from build123d import *

# Parameters (mm, degrees)
F0_W     = 37
F0_H     = 10
F0_R     = 1.5
F1_DEPTH = 11
F2_W     = 3.5
F2_H     = 11
F3_DEPTH = 16
F4_W     = 28
F4_H     = 10
F5_DEPTH = 6
F6_DEPTH = 7.5
F7_DEPTH = 7.5
F8_R     = 1
F9_DEPTH = 4
F10_R    = 5.2
F11_R    = 5.7


with BuildPart() as f1:
    # F0 (on Front) → F1 (new body)
    with BuildSketch(Plane.XZ):
        with Locations((-18.5, 5)):
            Rectangle(F0_W, F0_H)
        with Locations((-13.5, 5)):
            Circle(F0_R, mode=Mode.SUBTRACT)
        with Locations((-5, 5)):
            Circle(F0_R, mode=Mode.SUBTRACT)
    extrude(amount=-F1_DEPTH)

    # F2 (on face) → F3 (join)
    with BuildSketch(Plane.XY.offset(10)):
        with Locations((-35.25, 5.5)):
            Rectangle(F2_W, F2_H)
    extrude(amount=F3_DEPTH)

    # F4 (on face) → F5 (cut)
    with BuildSketch(Plane(origin=(0, 11, 0), x_dir=(-1, 0, 0), z_dir=(0, 1, 0))):
        with Locations((14, 5)):
            Rectangle(F4_W, F4_H)
        Polygon((6.5877132403, 7.75), (8.1754264805, 5), (6.5877132403, 2.25), (3.4122867597, 2.25), (1.8245735195, 5), (3.4122867597, 7.75), align=None, mode=Mode.SUBTRACT)
        Polygon((16.6754264805, 5), (15.0877132403, 2.25), (11.9122867597, 2.25), (10.3245735195, 5), (11.9122867597, 7.75), (15.0877132403, 7.75), align=None, mode=Mode.SUBTRACT)
    extrude(amount=-F5_DEPTH, mode=Mode.SUBTRACT)

    # F6 (cut): a face of the model
    f6_faces = [f1.faces().sort_by_distance(p)[0] for p in [
        (-2.6911883006, 11, 3.6670069439),
    ]]
    extrude(f6_faces, amount=-F6_DEPTH, mode=Mode.SUBTRACT)

    # F7 (cut): a face of the model
    f7_faces = [f1.faces().sort_by_distance(p)[0] for p in [
        (-13.5, 11, 7.6659861123),
    ]]
    extrude(f7_faces, amount=-F7_DEPTH, mode=Mode.SUBTRACT)

    # F8 (on face) → F9 (cut)
    with BuildSketch(Plane(origin=(-37, 0, 0), x_dir=(0, -1, 0), z_dir=(-1, 0, 0))):
        with Locations((-8.6, 2)):
            Circle(F8_R)
        with Locations((-2.4, 2)):
            Circle(F8_R)
        with Locations((-2.4, 4.8)):
            Circle(F8_R)
        with Locations((-8.6, 4.8)):
            Circle(F8_R)
        with Locations((-2.4, 7.6)):
            Circle(F8_R)
        with Locations((-8.6, 7.6)):
            Circle(F8_R)
        with Locations((-2.4, 10.4)):
            Circle(F8_R)
        with Locations((-8.6, 10.4)):
            Circle(F8_R)
        with Locations((-2.4, 13.2)):
            Circle(F8_R)
        with Locations((-8.6, 13.2)):
            Circle(F8_R)
        with Locations((-2.4, 16)):
            Circle(F8_R)
        with Locations((-8.6, 16)):
            Circle(F8_R)
        with Locations((-2.4, 18.8)):
            Circle(F8_R)
        with Locations((-8.6, 18.8)):
            Circle(F8_R)
        with Locations((-2.4, 21.6)):
            Circle(F8_R)
        with Locations((-8.6, 21.6)):
            Circle(F8_R)
        with Locations((-2.4, 24.4)):
            Circle(F8_R)
        with Locations((-8.6, 24.4)):
            Circle(F8_R)
    extrude(amount=-F9_DEPTH, mode=Mode.SUBTRACT)

    # F10
    f10_edges = [f1.edges().sort_by_distance(p)[0] for p in [
        (-28, 5, 5),
    ]]
    fillet(f10_edges, radius=F10_R)

    # F11
    f11_edges = [f1.edges().sort_by_distance(p)[0] for p in [
        (-28, 11, 5),
    ]]
    fillet(f11_edges, radius=F11_R)


solid = f1.part
The model under review builds one solid part; all positions refer to its coordinate system, in mm. A direction names the side the tool comes from. Round coordinates to 2 decimals unless told otherwise and drop trailing zeros. Loops run counter-clockwise (first coordinate to the right, second up) from the corner with the lowest first, then second, coordinate; pieces in that order, holes last. Notation, with made-up numbers: M 46.5,60 L 77.5,60 A20 ccw 77.5,89 Z; hole C -22,-33 d3. An arc over 180 degrees is marked long. Answer as a JSON object with one key per item and string values.
Item 1: Tool access review of faces 4 (the face through (-15, 2, 5)), 5 (the face through (-35.028, 1.476, 7.217)), 6 (the face through (-11.11, 4.26, 6.36)): name each direction out of +Z, -Z, +X, -X, +Y, -Y from which nothing blocks a thin tool from reaching the whole face with its end or side.
Check sheet entries:
{"face 4": "+Y, -Y", "face 5": "-X", "face 6": "+Y"}
Item 2: We need section B-B, the plane x = -13.5. State the section outline as (y, z) points, and give its area (4 significant figures).
Check sheet entries:
{"outline": "M 0,0 L 5,0 L 5,2.25 L 3.5,2.25 L 3.5,3.5 L 0,3.5 Z; M 0,6.5 L 3.5,6.5 L 3.5,7.75 L 5,7.75 L 5,10 L 0,10 Z", "area": "31.25 mm2"}
Item 3: The part is to be moulded in two halves that separate along Y. For faces 1 (the face through (-7.37, 4.26, 6.394)), 2 (the face through (-11, 5, 7)), 3 (the face through (-35.03, 1.86, 5.64)), say which applies: +Y half, -Y half, draft (parallel to the pull), parting line (faces both ways), or undercut.
Check sheet entries:
{"face 1": "draft", "face 2": "+Y half", "face 3": "undercut"}
Item 4: Clearance check with flat-ended pins moving along their axes: P1, Ø4, axis at x = -32.5, y = 8.5, coming from the -Z side; P2, Ø1.8, axis at y = 8.6, z = 24.4, coming from the +X side; P3, Ø1, axis at y = 8.5, z = 5, coming from the -X side; P4, Ø10, axis at x = -12, z = 6, coming from the +Y side. State where each tip first meets the part, or that it passes through.
Check sheet entries:
{"P1": "z = 0", "P2": "through", "P3": "x = -33", "P4": "y = 5"}
Item 5: We need section C-C, the plane y = 1. State the section outline as (x, z) points, and give its area (3 significant figures).
Check sheet entries:
{"outline": "M -37,0 L 0,0 L 0,10 L -33.5,10 L -33.5,26 L -37,26 Z; hole C -13.5,5 d3; hole C -5,5 d3", "area": "412 mm2"}
Item 6: For line 1 along Y through (x, z) = (-34.6, 10.4); line 2 along Z through (x, y) = (-22, 4); line 3 along X through (y, z) = (6, 11), list the stretches that pass through material, from the lowest coordinate up.
Check sheet entries:
{"line 1": "0 to 1.4, 3.4 to 7.6, 9.6 to 11", "line 2": "0 to 10", "line 3": "-37 to -33.5"}
Item 7: We need section A-A, the plane z = 16. State the section outline as (x, y) points, and give its area (3 significant figures).
Check sheet entries:
{"outline": "M -37,0 L -33.5,0 L -33.5,1.4 L -37,1.4 Z; M -37,3.4 L -33.5,3.4 L -33.5,7.6 L -37,7.6 Z; M -37,9.6 L -33.5,9.6 L -33.5,11 L -37,11 Z", "area": "24.5 mm2"}
Item 8: We need section D-D, the plane x = -22. State the section outline as (y, z) points, and give its area (3 significant figures).
Check sheet entries:
{"outline": "M 0,0 L 5,0 L 5,10 L 0,10 Z", "area": "50.0 mm2"}
